Geometry: final body of the model. Coordinates: model frame, mm. Face numbers are marked on the shaded views. A direction names the side the tool comes from. Give positions to 0.01 mm unless a question says otherwise; leave off trailing zeros. Order: outer loops, then holes, each group sorted by start corner. A loop starts at its lowest first (then second) coordinate and runs counter-clockwise, first axis right, second up. Notation, with made-up numbers: (12.25, 3) -> (63.25, 3) arc R19 cw to (63.25, 28) -> close; hole circle Ø2 at (73.25, -9.5). An arc over 180 degrees is marked (long way). One line per item, written item: value. Start each with the question number.
```python
from build123d import *

# Parameters (mm, degrees)
F2_SIZE = 1
F3_SIZE = 0.5


with BuildPart() as f1:
    # F0 (on Front) → F1 (revolve)
    with BuildSketch(Plane.XZ):
        Polygon((10, 30), (0, 30), (0, -20), (5, -20), (5, 0), (10, 0), align=None)
    revolve(axis=Axis((0, 0, 5), (0, 0, -1)))

    # F2
    f2_edges = [f1.edges().sort_by_distance(p)[0] for p in [
        (-10, 0, 30),
        (-5, 0, -20),
    ]]
    chamfer(f2_edges, length=F2_SIZE)

    # F3
    f3_edges = [f1.edges().sort_by_distance(p)[0] for p in [
        (-10, 0, 0),
    ]]
    chamfer(f3_edges, length=F3_SIZE)


solid = f1.part
```
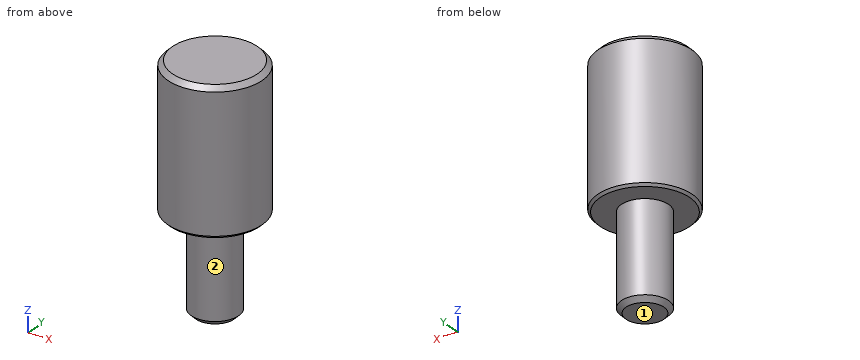
1. Cut plane C-C, the plane z = 16.5. Return loops of the section in (x, y).
2. Access query for the marked faces 1 and 2. Directions: +Z, -Z, +X, -X, +Y, -Y. A direction counts if a zero-diameter tool reaches every point of the face in a straight line with its end or side. Return the directions, or none.
3. Pin query (flat end, axial travel): P1, Ø5, axis at x = -4.5, z = 1, coming from the +Y side; P2, Ø10, axis at x = 6.5, z = 10, coming from the +Y side; P3, Ø3, axis at x = 7, z = 14, coming from the -Y side. Return the tip coordinate at first contact, or that it passes through.
4. Material intervals for L1, parallel to Z at x = -2.5, y = -5.25; L2, parallel to Y at x = -3, z = -6.5; L3, parallel to X at y = -1.25, z = -2, sorted ascending. Write a range as [from, to].
5. Cut plane A-A, the plane x = 0. Return loops of the section in (y, z).
Answers follow:
1. outline: circle Ø20 at (0, 0)
2. face 1: -Z, +X, -X, +Y, -Y
2. face 2: -Z
3. P1: stops at y = 9.8
3. P2: stops at y = 9.89
3. P3: stops at y = -8.35
4. L1: z = [0, 30]
4. L2: y = [-4, 4]
4. L3: x = [-4.84, 4.84]
5. outline: (-10, 0.5) -> (-9.5, 0) -> (-5, 0) -> (-5, -19) -> (-4, -20) -> (4, -20) -> (5, -19) -> (5, 0) -> (9.5, 0) -> (10, 0.5) -> (10, 29) -> (9, 30) -> (-9, 30) -> (-10, 29) -> close
